```python
from build123d import *

# Parameters (mm, degrees)
SKETCH_1_W          = 10
SKETCH_1_H          = 10
SKETCH_1_W_2        = 8
SKETCH_1_H_2        = 8
EXTRUDE_1_DEPTH     = 86
SKETCH_2_R          = 1.5
CUT_EXTRUDE_1_DEPTH = 11
CUT_EXTRUDE_2_DEPTH = 10


with BuildPart() as part:
    # 草图1 → 拉伸-薄壁1 (new body)
    with BuildSketch(Plane.XY):
        Rectangle(SKETCH_1_W, SKETCH_1_H)
        Rectangle(SKETCH_1_W_2, SKETCH_1_H_2, mode=Mode.SUBTRACT)
    extrude(amount=EXTRUDE_1_DEPTH)

    # 草图2 → 切除-拉伸1 (cut, through all)
    with BuildSketch(Plane(origin=(0, 5, 0), x_dir=(1, 0, 0), z_dir=(0, 1, 0))):
        with Locations((0, -54)):
            Circle(SKETCH_2_R)
        with Locations((0, -32)):
            Circle(SKETCH_2_R)
        with Locations((0, -43)):
            Circle(SKETCH_2_R)
        with Locations((0, -81)):
            Circle(SKETCH_2_R)
        with Locations((0, -5)):
            Circle(SKETCH_2_R)
    extrude(amount=-CUT_EXTRUDE_1_DEPTH, mode=Mode.SUBTRACT)

    # 草图3 → 切除-拉伸2 (cut)
    with BuildSketch(Plane(origin=(5, 0, 0), x_dir=(0, 0, -1), z_dir=(1, 0, 0))):
        Polygon((-86, 5), (-76, -5), (-86, -5), align=None)
        Polygon((0, 5), (-10, -5), (0, -5), align=None)
    extrude(amount=-CUT_EXTRUDE_2_DEPTH, mode=Mode.SUBTRACT)


solid = part.part
```
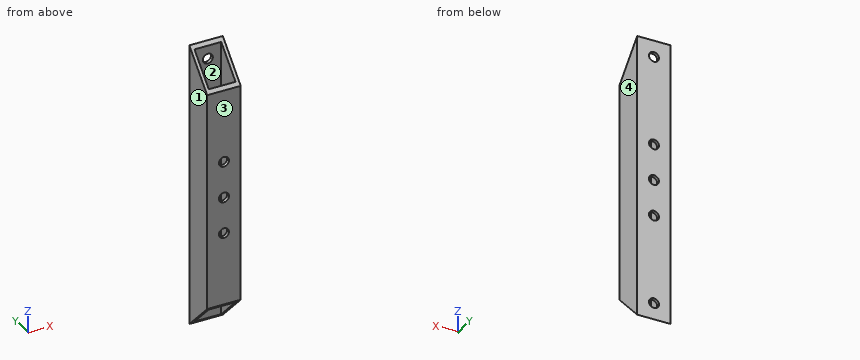
For this review, take the finished solid that the model builds, in its own axes (mm). Face numbers are marked on the shaded views. Round coordinates to 2 decimals unless told otherwise and drop trailing zeros. Write each loop counter-clockwise with the first axis right and the second up, starting at its lowest first coordinate (ties: lowest second). Pieces come first, ordered by that corner, then holes. Notation, with made-up numbers: (31.25, -8.5) -> (78.25, -8.5) arc R14 cw to (78.25, -0.5) -> close; hole circle Ø6 at (44, -31.5). An arc over 180 degrees is marked (long way). One line per question, with ' | ' between items. Start each with the question number.
1) Mouldability with a two-part tool opening along X and no side actions: class the marked faces 1, 2, 3 and 4 as +X half, -X half, draft (parallel to the pull), parting line (faces both ways), or undercut.
2) Add section C-C (z = 54). Write out the cut boundary in (x, y).
3) Add section A-A (z = 25.5). Write out the cut boundary in (x, y).
4) Add section D-D (z = 7.5). Write out the cut boundary in (x, y), and give its area (3 significant figures).
5) For pin 1 Ø2.5 at (x, z) = (0, 81) entering from +Y, flat-tipped, find the tip position at first contact; note if it passes through.
6) Wall thickness on line 1 along X through (y, z) = (4.85, 5); line 2 along Y through (x, z) = (1.75, 12.5): over which ranges is each line inside the solid? List them lowest first.
7) Add section B-B (y = -1.25). Write out the cut boundary in (x, z), and give its area (3 significant figures).
Reported:
1) face 1: -X half | face 2: undercut | face 3: draft | face 4: +X half
2) outline: (-5, -5) -> (-1.5, -5) -> (-1.5, -4) -> (-4, -4) -> (-4, 4) -> (-1.5, 4) -> (-1.5, 5) -> (-5, 5) -> close; (1.5, -5) -> (5, -5) -> (5, 5) -> (1.5, 5) -> (1.5, 4) -> (4, 4) -> (4, -4) -> (1.5, -4) -> close
3) outline: (-5, -5) -> (5, -5) -> (5, 5) -> (-5, 5) -> close; hole (-4, -4) -> (4, -4) -> (4, 4) -> (-4, 4) -> close
4) outline: (-5, -2.5) -> (-4, -2.5) -> (-4, 4) -> (4, 4) -> (4, -2.5) -> (5, -2.5) -> (5, 5) -> (-5, 5) -> close | area: 23.0 mm²
5) pin 1: passes through
6) line 1: x = -5 to -1.5, 1.5 to 5 | line 2: y = -5 to -4, 4 to 5
7) outline: (-5, 6.25) -> (-4, 6.25) -> (-4, 79.75) -> (-5, 79.75) -> close; (4, 6.25) -> (5, 6.25) -> (5, 79.75) -> (4, 79.75) -> close | area: 147 mm²
